```python
from build123d import *

# Parameters (mm, degrees)
SKETCH1_W           = 76.2
SKETCH1_H           = 12.7
BOSS_EXTRUDE1_DEPTH = 12.7
SKETCH3_R           = 1.25
CUT_EXTRUDE1_DEPTH  = 15.24
CUT_EXTRUDE2_START  = -15.24
SKETCH2_R           = 1.25
CUT_EXTRUDE2_DEPTH  = 15.24


with BuildPart() as part:
    # Sketch1 → Boss-Extrude1 (new body)
    with BuildSketch(Plane(origin=(0, 0, 0), x_dir=(1, 0, 0), z_dir=(0, 1, 0))):
        with Locations((38.1, 6.35)):
            Rectangle(SKETCH1_W, SKETCH1_H)
    extrude(amount=BOSS_EXTRUDE1_DEPTH)

    # Sketch3 → Cut-Extrude1 (cut)
    with BuildSketch(Plane.ZY):
        with Locations((-6.35, 6.35)):
            Circle(SKETCH3_R)
    extrude(amount=-CUT_EXTRUDE1_DEPTH, mode=Mode.SUBTRACT)

    # Sketch2 → Cut-Extrude2 (cut)
    with BuildSketch(Plane(origin=(76.2, 0, 0), x_dir=(0, 0, -1), z_dir=(1, 0, 0)).offset(CUT_EXTRUDE2_START)):
        with Locations(Location((6.35, 6.35, 0), (0, 0, 180))):
            Circle(SKETCH2_R)
    extrude(amount=CUT_EXTRUDE2_DEPTH, mode=Mode.SUBTRACT)


solid = part.part
```
Input: part model. Units: mm. Frame: model coordinates. A direction names the side the tool comes from. Coordinates: 2 decimals unless noted, no trailing zeros. Loops run counter-clockwise (first coordinate to the right, second up) from the corner with the lowest first, then second, coordinate; pieces in that order, holes last. Notation, with made-up numbers: (21.5, -9.75) - (63.5, -9.75) arc R7 cw to (63.5, -3.75) - close; hole circle Ø6 at (84.5, -31.75). An arc over 180 degrees is marked (long way). Answer in a Markdown table with one row per item.
(1) Set-up query: faces 4 (the face through (38, 6, -12.7)), 5 (the face through (15.24, 6, -6)), 6 (the face through (68.473, 5.505, -7.271)). Return all of +Z, -Z, +X, -X, +Y, -Y with unobstructed straight access to the full face (end or side cutting, diameter ignored); none if empty.
Model answer:
| item | result |
|---|---|
| face 4 | -Z, +X, -X, +Y, -Y |
| face 5 | -X |
| face 6 | +X |
(2) Pin query (flat end, axial travel): P1, Ø2, axis at y = 7, z = -6, coming from the +X side; P2, Ø2, axis at y = 6.35, z = -6.35, coming from the +X side. Return the tip coordinate at first contact, or that it passes through.
Model answer:
| item | result |
|---|---|
| P1 | stops at x = 76.2 |
| P2 | stops at x = 60.96 |
(3) Cut plane A-A on x = 9.5. Output: boundary loops of the cut face in (y, z), plus the area to 3 significant figures.
Model answer:
| item | result |
|---|---|
| outline | (0, -12.7) - (12.7, -12.7) - (12.7, 0) - (0, 0) - close; hole circle Ø2.5 at (6.35, -6.35) |
| area | 156 mm² |
(4) Cut plane B-B on z = -6.35. Output: boundary loops of the cut face in (x, y).
Model answer:
| item | result |
|---|---|
| outline | (0, 0) - (76.2, 0) - (76.2, 5.1) - (60.96, 5.1) - (60.96, 7.6) - (76.2, 7.6) - (76.2, 12.7) - (0, 12.7) - (0, 7.6) - (15.24, 7.6) - (15.24, 5.1) - (0, 5.1) - close |
(5) Mould query, pull axis Y, two halves, no side actions, for faces 1 (the face through (0, 6, -8)), 2 (the face through (7.513, 7.195, -7.271)), 3 (the face through (38, 0, -6)). Classes: pulls with the +Y half, pulls with the -Y half, needs draft (parallel to the pull), parting line crosses it, or undercut.
Model answer:
| item | result |
|---|---|
| face 1 | needs draft |
| face 2 | undercut |
| face 3 | pulls with the -Y half |
(6) Cut plane C-C on y = 6.35. Output: boundary loops of the cut face in (x, z).
Model answer:
| item | result |
|---|---|
| outline | (0, -12.7) - (76.2, -12.7) - (76.2, -7.6) - (60.96, -7.6) - (60.96, -5.1) - (76.2, -5.1) - (76.2, 0) - (0, 0) - (0, -5.1) - (15.24, -5.1) - (15.24, -7.6) - (0, -7.6) - close |
(7) Material intervals for L1, parallel to Y at x = 70.5, z = -6.35; L2, parallel to Z at x = 72.75, y = 6.35, sorted ascending. Write a range as from..to.
Model answer:
| item | result |
|---|---|
| L1 | y = 0..5.1, 7.6..12.7 |
| L2 | z = -12.7..-7.6, -5.1..0 |
